CAD build for the part. Positions are in the model's coordinates, mm. Face numbers are marked on the shaded views. A direction names the side the tool comes from. Coordinates: 2 decimals unless noted, no trailing zeros. Loops run counter-clockwise (first coordinate to the right, second up) from the corner with the lowest first, then second, coordinate; pieces in that order, holes last.
1) Saw through at A-A, the plane z = 1. Write the cut outline in (x, y), and give its area (3 significant figures).
2) Saw through at B-B, the plane y = 0. Write the cut outline in (x, z), and give its area (3 significant figures).
3) Pin check, flat tip, straight feed: pin 1 Ø0.8 at (y, z) = (0, -0.5) entering from +X. Stop position of the tip, or through.
4) Saw through at D-D, the plane y = -3.75. Write the cut outline in (x, z).
5) Wall check: line 1 along Y through (x, z) = (0, 1.6); line 2 along X through (y, z) = (0, 1.4); line 3 along X through (y, z) = (0, -0.3). Give the ranges that are in metal, low to high.
6) Saw through at C-C, the plane x = 0. Write the cut outline in (y, z).
7) Which spindle directions (+Z, -Z, +X, -X, +Y, -Y) get a long thin tool onto all of the face, cutting with end or side? Do the marked faces 1, 2 and 3. Say none if no direction does.
Autodesk Inventor part; units mm, degrees
ref_plane "YZ Plane" through (0, 0, 0) normal (1, 0, 0) x (0, 1, 0)
ref_plane "XZ Plane" through (0, 0, 0) normal (0, 1, 0) x (-1, 0, 0)
ref_plane "XY Plane" through (0, 0, 0) normal (0, 0, 1) x (1, 0, 0)
sketch "Sketch1" plane through (0, 0, 0) normal (0, 0, 1) x (1, 0, 0)
  line L0 (22.8551, 4.5234) -> (0.5229, 6.4772)
  arc A0 (0.5229, 6.4772) -> (-0.5229, 6.4772) centre (0, 0.5) ccw
  line L1 (-0.5229, 6.4772) -> (-22.8551, 4.5234)
  arc A1 (-22.8551, 4.5234) -> (-22.8551, -4.5234) centre (-22.4594, 0) ccw
  line L2 (-22.8551, -4.5234) -> (-0.5229, -6.4772)
  arc A2 (-0.5229, -6.4772) -> (0.5229, -6.4772) centre (0, -0.5) ccw
  line L3 (0.5229, -6.4772) -> (22.8551, -4.5234)
  arc A3 (22.8551, -4.5234) -> (22.8551, 4.5234) centre (22.4594, 0) ccw
  circle A4 centre (0, 0) radius 2.5
  dimension "d0" = 54
  dimension "d1" = 13
  dimension "d2" = 5
  dimension "d4" = 6
  dimension "d11" = 10
extrude "Extrusion1" add sketch "Sketch1" along normal blind 2
sketch "Sketch2" plane through (0, 0, 0) normal (0, 0, -1) x (-1, 0, 0)
  arc A0 (0.5229, 6.4772) -> (-0.5229, 6.4772) centre (0, 0.5) ccw
  line L0 (-22.8551, 4.5234) -> (-0.5229, 6.4772)
  arc A1 (-22.8551, 4.5234) -> (-22.8551, -4.5234) centre (-22.4594, 0) ccw construction
  line L1 (-0.5229, -6.4772) -> (-22.8551, -4.5234)
  arc A2 (-0.5229, -6.4772) -> (0.5229, -6.4772) centre (0, -0.5) ccw
  line L2 (22.8551, -4.5234) -> (0.5229, -6.4772)
  arc A3 (22.8551, -4.5234) -> (22.8551, 4.5234) centre (22.4594, 0) ccw construction
  line L3 (0.5229, 6.4772) -> (22.8551, 4.5234)
  circle A4 centre (0, 0) radius 2.5
  line L4 (-9, 5.7355) -> (-9, -5.7355)
  line L5 (-22.8551, 4.5234) -> (-0.5229, 6.4772) construction
  line L6 (9, 5.7355) -> (9, -5.7355)
  line L7 (0.5229, 6.4772) -> (22.8551, 4.5234) construction
  point P0 (9, 5.7355)
  dimension "d7" = 18
  dimension "d8" = 9
extrude "Extrusion2" add sketch "Sketch2" along normal blind 1
properties part number "NyArm"
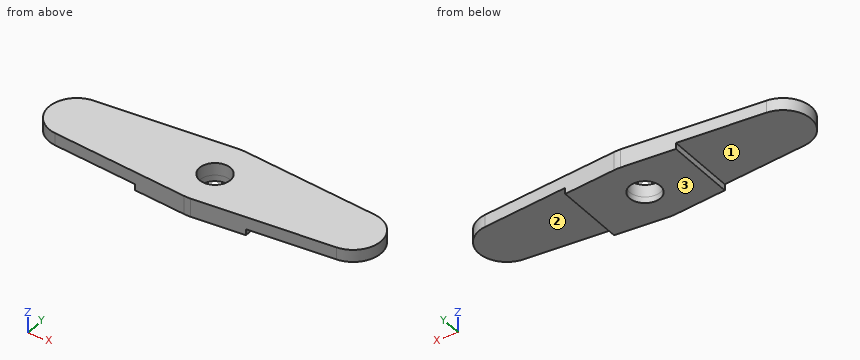
Data:
1. outline: (-22.86, -4.52) - (-0.52, -6.48) arc R6 ccw to (0.52, -6.48) - (22.86, -4.52) arc R4.54 ccw to (22.86, 4.52) - (0.52, 6.48) arc R6 ccw to (-0.52, 6.48) - (-22.86, 4.52) arc R4.54 ccw to start; hole circle Ø5 at (0, 0)
1. area: 543 mm2
2. outline: (-27, 0) - (-9, 0) - (-9, -1) - (-2.5, -1) - (-2.5, 2) - (-27, 2) - close; (2.5, -1) - (9, -1) - (9, 0) - (27, 0) - (27, 2) - (2.5, 2) - close
2. area: 111 mm2
3. pin 1: stops at x = 9
4. outline: (-25.02, 0) - (-9, 0) - (-9, -1) - (9, -1) - (9, 0) - (25.02, 0) - (25.02, 2) - (-25.02, 2) - close
5. line 1: y = -6.5 to -2.5, 2.5 to 6.5
5. line 2: x = -27 to -2.5, 2.5 to 27
5. line 3: x = -9 to -2.5, 2.5 to 9
6. outline: (-6.5, -1) - (-2.5, -1) - (-2.5, 2) - (-6.5, 2) - close; (2.5, -1) - (6.5, -1) - (6.5, 2) - (2.5, 2) - close
7. face 1: -Z, -X, +Y, -Y
7. face 2: -Z, +X, +Y, -Y
7. face 3: -Z, +X, -X, +Y, -Y
